Verification items for the finished model (mm, model axes). A direction names the side the tool comes from. Give positions to 0.01 mm unless a question says otherwise; leave off trailing zeros. Write each loop counter-clockwise with the first axis right and the second up, starting at its lowest first coordinate (ties: lowest second). Pieces come first, ordered by that corner, then holes. Notation, with made-up numbers: M 86,-14 L 113,-14 A27 cw 113,22 Z; hole C 69.25,-30.5 d1. An arc over 180 degrees is marked long. Write item = value, one per line.
from build123d import *

# Parameters (mm, degrees)
F0_W      = 129.54
F0_H      = 85.09
F1_DEPTH  = 3.175
F2_W      = 129.54
F2_H      = 85.09
F2_W_2    = 124.46
F2_H_2    = 80.01
F3_DEPTH  = 12.7
F4_R      = 9.525
F5_SIZE   = 2.54
F2_R      = 4.191
F2_R_2    = 2.286
F6_DEPTH  = 12.7
F2_R_3    = 3.302
F7_DEPTH  = 12.7
F9_R      = 2.2225
F10_DEPTH = 10.16
F8_R      = 2.2225
F11_DEPTH = 10.16
F13_W     = 22.86
F13_H     = 5.08
F14_DEPTH = 2.54
F12_W     = 43.18
F12_H     = 11.43
F15_DEPTH = 3.811
F16_SIZE  = 0.635
F17_SIZE  = 0.635


with BuildPart() as f1:
    # F0 (on Top) → F1 (new body)
    with BuildSketch(Plane.XY):
        Rectangle(F0_W, F0_H)
    extrude(amount=F1_DEPTH)

    # F2 (on face) → F3 (join)
    with BuildSketch(Plane.XY.offset(3.175)):
        Rectangle(F2_W, F2_H)
        Rectangle(F2_W_2, F2_H_2, mode=Mode.SUBTRACT)
    extrude(amount=F3_DEPTH)

    # F4
    f4_edges = [f1.edges().sort_by_distance(p)[0] for p in [
        (62.23, 40.005, 9.525),
        (62.23, -40.005, 9.525),
        (-62.23, -40.005, 9.525),
        (-62.23, 40.005, 9.525),
        (64.77, 42.545, 7.9375),
        (64.77, -42.545, 7.9375),
        (-64.77, -42.545, 7.9375),
        (-64.77, 42.545, 7.9375),
    ]]
    fillet(f4_edges, radius=F4_R)

    # F5
    f5_edges = [f1.edges().sort_by_distance(p)[0] for p in [
        (0, 40.005, 3.175),
        (0, 42.545, 0),
    ]]
    chamfer(f5_edges, length=F5_SIZE)

    # F2 (on face) → F6 (join)
    with BuildSketch(Plane.XY.offset(3.175)):
        with Locations((-54.9275, -33.909)):
            Circle(F2_R)
        with Locations((-54.9275, -33.909)):
            Circle(F2_R_2, mode=Mode.SUBTRACT)
        with Locations((54.9275, -33.909)):
            Circle(F2_R)
        with Locations((54.9275, -33.909)):
            Circle(F2_R_2, mode=Mode.SUBTRACT)
    extrude(amount=F6_DEPTH)

    # F2 (on face) → F7 (join)
    with BuildSketch(Plane.XY.offset(3.175)):
        with Locations((-54.9275, 33.909)):
            Circle(F2_R_3)
        with Locations((54.9275, 33.909)):
            Circle(F2_R_3)
    extrude(amount=F7_DEPTH)

    # F9 (on face) → F10 (join)
    with BuildSketch(Plane.XY.offset(15.875)):
        with Locations((-54.9275, 33.909)):
            Circle(F9_R)
    extrude(amount=F10_DEPTH)

    # F8 (on face) → F11 (join)
    with BuildSketch(Plane.XY.offset(15.875)):
        with Locations((54.9275, 33.909)):
            Circle(F8_R)
    extrude(amount=F11_DEPTH)

    # F13 (on face) → F14 (cut, through all)
    with BuildSketch(Plane.XZ.offset(42.545)):
        with Locations((1.905, 13.335)):
            Rectangle(F13_W, F13_H)
    extrude(amount=-F14_DEPTH, mode=Mode.SUBTRACT)

    # F12 (on face) → F15 (cut, through all)
    with BuildSketch(Plane(origin=(-64.77, 0, 0), x_dir=(0, -1, 0), z_dir=(-1, 0, 0))):
        with Locations((7.62, 10.16)):
            Rectangle(F12_W, F12_H)
    extrude(amount=-F15_DEPTH, mode=Mode.SUBTRACT)

    # F16
    f16_edges = [f1.edges().sort_by_distance(p)[0] for p in [
        (-57.15, 33.909, 26.035),
    ]]
    chamfer(f16_edges, length=F16_SIZE)

    # F17
    f17_edges = [f1.edges().sort_by_distance(p)[0] for p in [
        (52.705, 33.909, 26.035),
    ]]
    chamfer(f17_edges, length=F17_SIZE)


solid = f1.part
1) Material ranges on probe 1 along Y at (x, z) = (17, 12.5) (3 decimals); probe 2 along Y at (x, z) = (54, 10.75) (3 decimals); probe 3 along X at (y, z) = (-30.5, 7), recorded low to high. Write a range as from..to.
From the geometry:
probe_1 = -42.545..-40.005, 40.005..42.545
probe_2 = -42.545..-39.917, -37.996..-35.998, -31.82..-29.822, 30.74..37.078, 39.917..42.545
probe_3 = -64.77..-62.23, -57.37..-52.49, 52.49..57.37, 62.23..64.77
2) Draft check along X on faces 1 (the flat face through (63.52, 0.46, 1.29)), 2 (the flat face through (-1, 40.005, 11)), 3 (the flat face through (-55, 34, 26.035)). Enter one of: +X half, -X half, draft (parallel to the pull), parting line (faces both ways), or undercut.
From the geometry:
face_1 = +X half
face_2 = undercut
face_3 = draft
3) Cross-section at B-B on z = 13. Count the separate pieces of the cut face and the enclosed holes in it, plus the area to 3 significant figures.
From the geometry:
separate_pieces = 6
enclosed_holes = 2
area = 1,040 mm^2
4) Tool access check on faces 4 (the flat face through (-55, -34, 3.175)), 5 (the flat face through (2, -41, 10.795)), 6 (the flat face through (-64.77, 7, 3)). Record the directions out of +Z, -Z, +X, -X, +Y, -Y that give a thin tool (end or side, any length) a straight path to the whole face; none if there is none.
From the geometry:
face_4 = +Z
face_5 = +Z, -Y
face_6 = +Z, -Z, -X, +Y, -Y
5) Depth check by flat-ended pin: P1, Ø0.8, axis at x = 5, y = -41.5, coming from the +Z side (3 decimals); P2, Ø1.3, axis at y = -41.5, z = 13, coming from the -X side; P3, Ø1.1, axis at x = -62.5, z = 10.5, coming from the +Y side. Enter the tip coordinate at first touch or a pass-through.
From the geometry:
P1 = 10.795
P2 = -60.67
P3 = 39.79
6) Cross-section at D-D on y = -14. Record the boundary of the cut face in (x, z) (3 decimals), plus the area to 3 significant figures.
From the geometry:
outline = M -64.77,2.54 L -62.23,0 L 62.23,0 L 64.77,2.54 L 64.77,15.875 L 62.23,15.875 L 62.23,5.715 L 59.69,3.175 L -59.69,3.175 L -60.96,4.445 L -64.77,4.445 Z
area = 446 mm^2
7) Cross-section at A-A on y = 27. Record the boundary of the cut face in (x, z) (3 decimals), plus the area to 3 significant figures.
From the geometry:
outline = M -64.77,2.54 L -62.23,0 L 62.23,0 L 64.77,2.54 L 64.77,15.875 L 62.23,15.875 L 62.23,5.715 L 59.69,3.175 L -59.69,3.175 L -62.23,5.715 L -62.23,15.875 L -64.77,15.875 Z
area = 476 mm^2
8) Cross-section at C-C on x = 4. Record the boundary of the cut face in (y, z) (3 decimals), plus the area to 3 significant figures.
From the geometry:
outline = M -42.545,2.54 L -40.005,0 L 40.005,0 L 42.545,2.54 L 42.545,15.875 L 40.005,15.875 L 40.005,5.715 L 37.465,3.175 L -37.465,3.175 L -40.005,5.715 L -40.005,10.795 L -42.545,10.795 Z
area = 322 mm^2
